The figure shows three views and two pictorial views of one solid part (mm, origin at its lowest corner). Answer the questions. A direction names the side the tool comes from. Coordinates: 2 decimals unless noted, no trailing zeros. Order: outer loops, then holes, each group sorted by start corner. A loop starts at its lowest first (then second) coordinate and runs counter-clockwise, first axis right, second up. Notation, with made-up numbers: M 67.25,85 L 102.25,85 A14 cw 102.25,89 Z; hole C 79.25,-0.75 d2. An arc over 180 degrees is marked long. Answer in a Markdown table with one row per item. Add a question column.
Item 1: The part is cut by section B-B (z = 8). Write down the section's boundary in (x, y).
Item 2: Which of the six approach directions +Z, -Z, +X, -X, +Y, -Y give full straight-line access (tool end or side, diameter ignored) to the marked faces 5 and 6?
Item 3: The part is cut by section A-A (x = 68). Write down the section's boundary in (y, z).
Item 4: The part is cut by section D-D (x = 2.54). Write down the section's boundary in (y, z).
Item 5: The part is cut by section C-C (y = 12.7). State how many separate pieces and enclosed holes the cut face has, then the cut area to 3 significant figures.
Item 6: The mould has two halves that part along Z. Classify the marked faces 1, 2, 3 and 4: released by +Z, released by -Z, zero draft, split by the parting line, or undercut.
Item 7: A flat-ended cylindrical pin translates along its axis: pin 1 Ø1 at (x, z) = (28, 22.5) entering from +Y. Find the tip coordinate at first contact, or state that the pin passes through.
Item 8: Consider line 1 (X direction, y = 1.2, z = 19.05); line 2 (Y direction, x = 25.4, z = 1.45); line 3 (Y direction, x = 2.54, z = 36.65). Determine where each line is inside the solid, lowest interval first. Write a range as from..to.
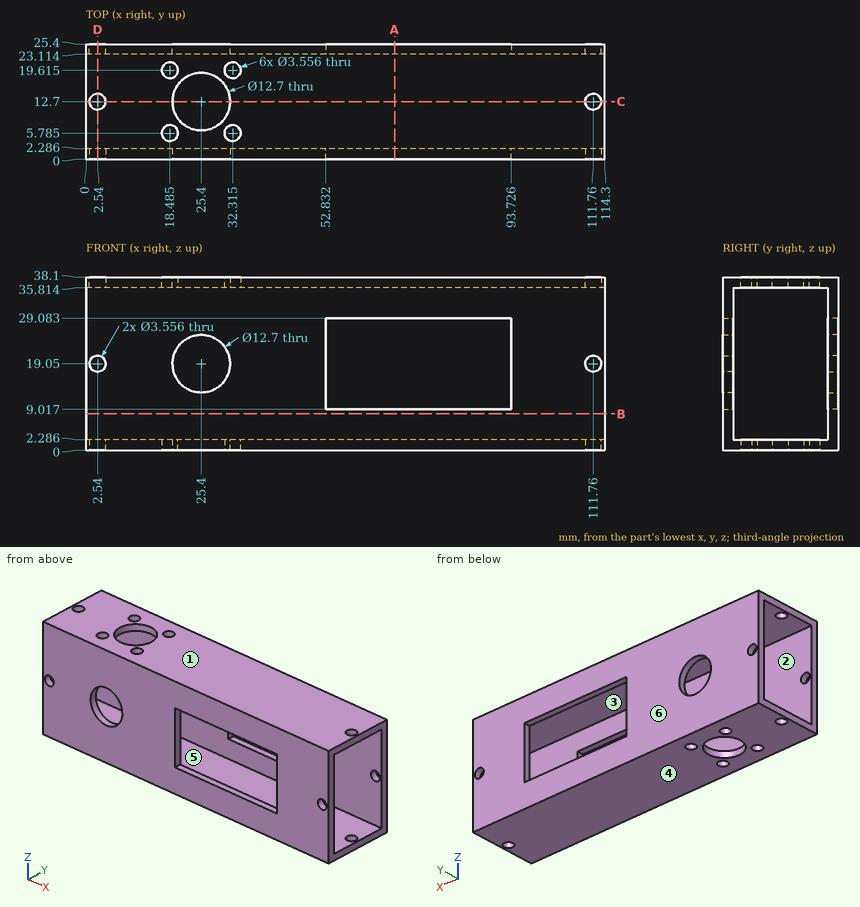
Reply:
| question | item | result |
|---|---|---|
| 1 | outline | M 0,0 L 114.3,0 L 114.3,2.29 L 0,2.29 Z; M 0,23.11 L 114.3,23.11 L 114.3,25.4 L 0,25.4 Z |
| 2 | face 5 | +X, -X |
| 2 | face 6 | +Z, -Z, +X, -X, +Y |
| 3 | outline | M 0,0 L 25.4,0 L 25.4,9.02 L 23.11,9.02 L 23.11,2.29 L 2.29,2.29 L 2.29,9.02 L 0,9.02 Z; M 0,29.08 L 2.29,29.08 L 2.29,35.81 L 23.11,35.81 L 23.11,29.08 L 25.4,29.08 L 25.4,38.1 L 0,38.1 Z |
| 4 | outline | M 0,0 L 10.92,0 L 10.92,2.29 L 2.29,2.29 L 2.29,17.27 L 0,17.27 Z; M 0,20.83 L 2.29,20.83 L 2.29,35.81 L 10.92,35.81 L 10.92,38.1 L 0,38.1 Z; M 14.48,0 L 25.4,0 L 25.4,17.27 L 23.11,17.27 L 23.11,2.29 L 14.48,2.29 Z; M 14.48,35.81 L 23.11,35.81 L 23.11,20.83 L 25.4,20.83 L 25.4,38.1 L 14.48,38.1 Z |
| 5 | separate pieces | 8 |
| 5 | enclosed holes | 0 |
| 5 | area | 432 mm2 |
| 6 | face 1 | released by +Z |
| 6 | face 2 | undercut |
| 6 | face 3 | undercut |
| 6 | face 4 | released by -Z |
| 7 | pin 1 | passes through |
| 8 | line 1 | x = 0..0.76, 4.32..19.05, 31.75..52.83, 93.73..109.98, 113.54..114.3 |
| 8 | line 2 | y = 0..6.35, 19.05..25.4 |
| 8 | line 3 | y = 0..10.92, 14.48..25.4 |
